from build123d import *

# Parameters (mm, degrees)
EXTRUDE_1_DEPTH     = 3
FILLET_1_R          = 1
SKETCH_2_R          = 1.55
CUT_EXTRUDE_1_DEPTH = 4


with BuildPart() as part:
    # Эскиз1 → Бобышка-Вытянуть1 (new body)
    with BuildSketch(Plane.XY):
        Polygon((34.9, -12), (34.9, 12), (34.9, 17.8), (21.1, 12), (-21.1, 12), (-34.9, 17.8), (-34.9, 12), (-34.9, -12), (-34.9, -17.8), (-21.1, -12), (21.1, -12), (34.9, -17.8), align=None)
    extrude(amount=EXTRUDE_1_DEPTH)

    # Скругление1
    fillet_1_edges = [part.edges().sort_by_distance(p)[0] for p in [
        (-34.9, 17.8, 1.5),
        (34.9, 17.8, 1.5),
        (34.9, -17.8, 1.5),
        (-34.9, -17.8, 1.5),
    ]]
    fillet(fillet_1_edges, radius=FILLET_1_R)

    # Эскиз2 → Вырез-Вытянуть1 (cut, through all)
    with BuildSketch(Plane.XY.offset(3)):
        with Locations((-24.25, 0)):
            Circle(SKETCH_2_R)
        with Locations((24.25, 0)):
            Circle(SKETCH_2_R)
    extrude(amount=-CUT_EXTRUDE_1_DEPTH, mode=Mode.SUBTRACT)


solid = part.part
Input: part model. Units: mm. Frame: model coordinates. A direction names the side the tool comes from. Give positions to 0.01 mm unless a question says otherwise; leave off trailing zeros. Write each loop counter-clockwise with the first axis right and the second up, starting at its lowest first coordinate (ties: lowest second). Pieces come first, ordered by that corner, then holes.
Q1. Section D-D, the plane x = 12. Output: boundary loops of the cut face in (y, z).
Q2. Section B-B, the plane z = 0.8. Output: boundary loops of the cut face in (x, y).
Q3. Section A-A, the plane y = 0. Output: boundary loops of the cut face in (x, z), plus the area to 3 significant figures.
Q4. Set-up query: faces 4 (the face through (34.9, 0, 1)), 5 (the face through (27.393, 14.645, 1.479)), 6 (the face through (27.219, -14.572, 1.479)). Return all of +Z, -Z, +X, -X, +Y, -Y with unobstructed straight access to the full face (end or side cutting, diameter ignored); none if empty.
Q5. Material intervals for probe 1 along X at (y, z) = (-0.5, 2.4); probe 2 along Y at (x, z) = (1.5, 1.15); probe 3 along Y at (x, z) = (-24.25, 2.15), sorted ascending.
Q6. First-contact query: P1, Ø1.9, axis at x = 24.25, y = 0, coming from the -Z side; P2, Ø1.5, axis at x = 19, z = 0.5, coming from the +Y side. Flat tips, straight axial feed; report the tip coordinate or a pass-through.
Q7. Section C-C, the plane x = 24.25. Output: boundary loops of the cut face in (y, z).
Q8. Pull-direction query (Y, two-part tool) for faces 1 (the face through (-22.818, -0.594, 1.521)), 2 (the face through (-27.393, -14.645, 1.479)), 3 (the face through (-34.9, 0, 1)); classes: pulls with the +Y half, pulls with the -Y half, needs draft (parallel to the pull), parting line crosses it, or undercut.
Filled in:
1. outline: (-12, 0) - (12, 0) - (12, 3) - (-12, 3) - close
2. outline: (-34.9, -16.29) arc R1 ccw to (-33.51, -17.22) - (-21.1, -12) - (21.1, -12) - (33.51, -17.22) arc R1 ccw to (34.9, -16.29) - (34.9, 16.29) arc R1 ccw to (33.51, 17.22) - (21.1, 12) - (-21.1, 12) - (-33.51, 17.22) arc R1 ccw to (-34.9, 16.29) - close; hole circle Ø3.1 at (-24.25, 0); hole circle Ø3.1 at (24.25, 0)
3. outline: (-34.9, 0) - (-25.8, 0) - (-25.8, 3) - (-34.9, 3) - close; (-22.7, 0) - (22.7, 0) - (22.7, 3) - (-22.7, 3) - close; (25.8, 0) - (34.9, 0) - (34.9, 3) - (25.8, 3) - close
3. area: 191 mm2
4. face 4: +Z, -Z, +X, +Y, -Y
4. face 5: +Z, -Z, +Y
4. face 6: +Z, -Z, -Y
5. probe 1: x = -34.9 to -25.72, -22.78 to 22.78, 25.72 to 34.9
5. probe 2: y = -12 to 12
5. probe 3: y = -13.32 to -1.55, 1.55 to 13.32
6. P1: passes through
6. P2: stops at y = 12
7. outline: (-13.32, 0) - (-1.55, 0) - (-1.55, 3) - (-13.32, 3) - close; (1.55, 0) - (13.32, 0) - (13.32, 3) - (1.55, 3) - close
8. face 1: undercut
8. face 2: pulls with the -Y half
8. face 3: needs draft
